Verification items for the finished model (mm, model axes). A direction names the side the tool comes from. Round coordinates to 2 decimals unless told otherwise and drop trailing zeros. Loops run counter-clockwise (first coordinate to the right, second up) from the corner with the lowest first, then second, coordinate; pieces in that order, holes last. Notation, with made-up numbers: (-31.75, 5) - (-19.75, 5) arc R30 ccw to (-19.75, 44) - close; hole circle Ø4 at (80.25, -3). An arc over 180 degrees is marked (long way). Use CSV: the item, a comma, the result in double quotes.
Autodesk Inventor part; units mm, degrees
ref_plane "Work Plane1" through (-14, 1, -1) normal (-1, 0, 0) x (0, 0, 1)
ref_plane "Work Plane2" through (0, 1, 0) normal (0, 1, 0) x (-1, 0, 0)
ref_plane "YZ Plane" through (0, 0, 0) normal (1, 0, 0) x (0, 1, 0)
sketch "Sketch1" plane through (0, 0, 0) normal (0, 1, 0) x (-1, 0, 0)
  line L0 (0, 0) -> (20, 0)
  line L1 (20, 0) -> (20, -2)
  line L2 (20, -2) -> (0, -2)
  line L3 (0, -2) -> (0, 0)
  dimension "d0" = 20
  dimension "d1" = 2
extrude "Extrusion1" add sketch "Sketch1" along normal blind 2
sketch "Sketch2" plane through (0, 2, 0) normal (0, 1, 0) x (1, 0, 0)
  line L0 (0, 2) -> (-20, 2)
  line L1 (0, 2) -> (0, 4)
  line L2 (0, 4) -> (2, 4)
  line L3 (2, 4) -> (2, -2)
  line L4 (2, -2) -> (0, -2)
  line L5 (0, 0) -> (0, 2)
  line L6 (0, -2) -> (0, 0)
  dimension "d4" = 2
  dimension "d5" = 2
  dimension "d6" = 6
extrude "Extrusion2" add sketch "Sketch2" against normal blind 2
sketch "Sketch3" plane through (0, 2, 0) normal (0, 1, 0) x (1, 0, 0)
  line L0 (0, 0) -> (0, -2)
  line L1 (0, -2) -> (0, -1)
  line L2 (2, 4) -> (2, -2)
  line L3 (2, -2) -> (2, -0.5)
  line L4 (2, -0.5) -> (1, -0.5)
  circle A0 centre (1, -0.5) radius 0.5
  line L5 (2, 1) -> (1.5, 1)
  circle A1 centre (1, 2.5) radius 0.5
  dimension "d9" = 1.5
  dimension "d10" = 1
  dimension "d11" = 1
extrude "Extrusion3" cut sketch "Sketch3" against normal blind 2
sketch "Sketch4" plane through (0, 2, -4) normal (-1, 0, 0) x (0, 0, 1)
  line L0 (2, 0) -> (4, 0)
  line L1 (3, 0) -> (3, -2)
  line L2 (2, -2) -> (4, -2)
  circle A0 centre (3, -1) radius 1
  line L3 (2, -2) -> (2, 0)
  circle A1 centre (3, -1) radius 1.4142
extrude "Extrusion4" cut sketch "Sketch4" along normal blind 100 contours L0 A0 L3 | L3 A1 | L0 A1 L2 A0 | A0 L2 L3
ref_plane "Work Plane1" through (-14, 1, -1) normal (-1, 0, 0) x (0, 0, 1)
sketch "Sketch5" plane through (-14, 1, -1) normal (-1, 0, 0) x (0, 0, 1)
  circle A0 centre (0, 0) radius 5
  point P0 (1, -1)
  dimension "d17" = 10
extrude "Extrusion5" add sketch "Sketch5" along normal mid plane 1
sketch "Sketch6" plane through (-20, 1, -1) normal (-1, 0, 0) x (0, 0, 1)
  circle A0 centre (0, 0) radius 5
  point P0 (1, -1)
extrude "Extrusion6" cut sketch "Sketch6" against normal blind 5.5
sketch "Sketch7" plane through (-13.5, 1, -1) normal (1, 0, 0) x (0, 0, -1)
  arc A0 (0, 1) -> (0, -1) centre (0, 0) ccw
  circle A1 centre (0, 0) radius 5
  point P0 (-1, -1)
extrude "Extrusion7" add sketch "Sketch7" along normal blind 14.5
sketch "Sketch8" plane through (1, 1, -1) normal (1, 0, 0) x (0, 0, -1)
  circle A0 centre (0, 0) radius 5
  point P0 (-1, -1)
extrude "Extrusion8" cut sketch "Sketch8" along normal blind 13.5
sketch "Sketch9" plane through (1, 1, -1) normal (1, 0, 0) x (0, 0, -1)
  point P0 (-1, -1)
sketch "Sketch10" plane through (1, 1, -1) normal (1, 0, 0) x (0, 0, -1)
  point P0 (-1, -1)
sketch "Sketch11" plane through (1, 1, -1) normal (1, 0, 0) x (0, 0, -1)
  line L0 (0, 0) -> (1.5, 0)
  line L1 (0, 0) -> (-1.5, 0)
  point P0 (-1, -1)
  dimension "d26" = 1.5
  dimension "d27" = 1.5
ref_plane "Work Plane2" through (0, 1, 0) normal (0, 1, 0) x (-1, 0, 0)
sketch "Sketch12" plane through (0, 1, 0) normal (0, 1, 0) x (-1, 0, 0)
  line L0 (-1, 4) -> (-1, -6)
  line L1 (-1, -1) -> (-1, 0)
  line L2 (-1, -1) -> (-1, -2)
  line L3 (-1, -2) -> (-2, -2)
  line L4 (-1, 0) -> (-2, 0)
  line L5 (-1, 0) -> (-1, -0.5)
  line L6 (-1, 0) -> (-1, 0.5)
  line L7 (-1, -2) -> (-1, -1.5)
  line L8 (-1, -2) -> (-1, -2.5)
  line L9 (-2, -2) -> (-1, -2.5)
  line L10 (-1, -1.5) -> (-2, -2)
  line L11 (-2, 0) -> (-1, -0.5)
  line L12 (-2, 0) -> (-1, 0.5)
  point P0 (0, 0)
  point P1 (-1, -0.5)
  dimension "d32" = 1
  dimension "d33" = 1
  dimension "d34" = 1
  dimension "d35" = 1
  dimension "d36" = 0.5
  dimension "d37" = 0.5
  dimension "d38" = 0.5
  dimension "d39" = 0.5
extrude "Extrusion9" add sketch "Sketch12" along normal mid plane 8
properties part number "drive_shaft_v2"
1) Cross-section at B-B, the plane z = -1. Record the cut outline in (x, y).
Returned:
outline,"(-14.5, -4) - (1, -4) - (1, 6) - (-14.5, 6) - close"
2) Thickness scan on probe 1 along X at (y, z) = (-0.5, -4.5); probe 2 along Y at (x, z) = (-1.75, 1.25); probe 3 along Y at (x, z) = (-6.75, 0.75). Record the ranges inside material, lowest first. Write a range as [from, to].
Returned:
probe 1,"x = [-14.5, 1]"
probe 2,"y = [-3.47, 5.47]"
probe 3,"y = [-3.68, 5.68]"
3) Cross-section at D-D, the plane y = -1.5. Record the cut outline in (x, z).
Returned:
outline,"(-14.5, -5.33) - (1, -5.33) - (1, -2.5) - (2, -2) - (1, -1.5) - (1, -0.5) - (2, 0) - (1, 0.5) - (1, 3.33) - (-14.5, 3.33) - close"
4) Access from +Z, -Z, +X, -X, +Y, -Y to the whole of each face (thin tool, end or side, straight path). Record for faces 1 (the face through (1.4, 5, -2)), 2 (the face through (1.507, 0.944, 0.247)), 3 (the face through (1.507, 0.944, -0.247)), 4 (the face through (1.4, -3, 0)).
Returned:
face 1,"+Z, -Z, +X, +Y"
face 2,"+Z, +X, +Y, -Y"
face 3,"+X, +Y, -Y"
face 4,"+Z, -Z, +X, -Y"
5) Gauge pin test, flat ends, axial feed: pin 1 Ø1.1 at (x, z) = (1.5, -2) entering from -Y; pin 2 Ø0.8 at (x, z) = (1.5, 0) entering from +Y; pin 3 Ø1.1 at (x, z) = (1.5, -2) entering from +Y. Record the tip position at first contact, or that the pin passes through.
Returned:
pin 1,"stops at y = -3.94"
pin 2,"stops at y = 5"
pin 3,"stops at y = 5.94"
6) Cross-section at A-A, the plane y = 1.5. Record the cut outline in (x, z).
Returned:
outline,"(-14.5, -5.97) - (1, -5.97) - (1, -2.5) - (2, -2) - (1, -1.5) - (1, -0.5) - (2, 0) - (1, 0.5) - (1, 3.97) - (-14.5, 3.97) - close"
7) Mould release check, pull along Z, two halves, no side actions. Record for faces 5 (the face through (-14.5, 1, -1)), 6 (the face through (1.507, 0.944, -2.247)), 7 (the face through (1.493, 0.944, -1.747)): +Z half, -Z half, draft (parallel to the pull), parting line (faces both ways), or undercut.
Returned:
face 5,"draft"
face 6,"-Z half"
face 7,"undercut"
8) Cross-section at C-C, the plane x = -3.5. Record the cut outline in (y, z).
Returned:
outline,"circle Ø10 at (1, -1)"
